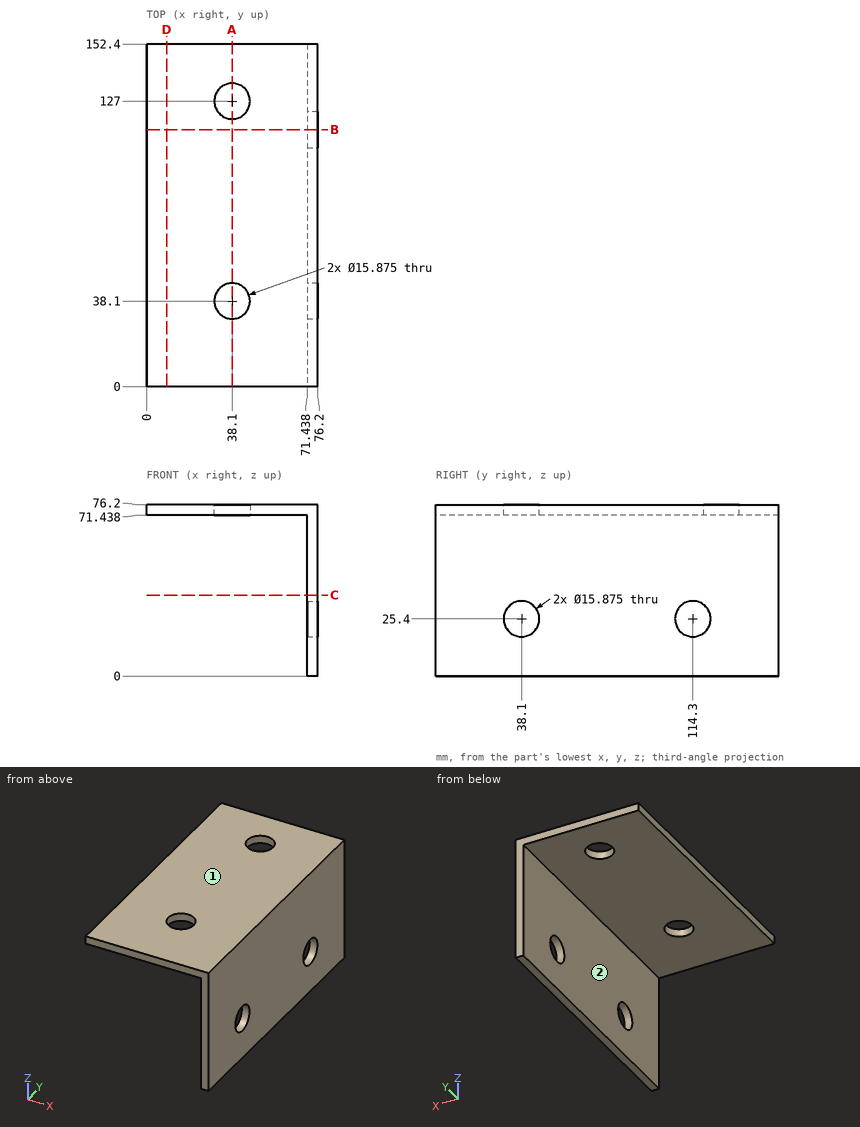
The figure shows three views and two pictorial views of one solid part (mm, origin at its lowest corner). Answer the questions. A direction names the side the tool comes from. Round coordinates to 2 decimals unless told otherwise and drop trailing zeros. Loops run counter-clockwise (first coordinate to the right, second up) from the corner with the lowest first, then second, coordinate; pieces in that order, holes last. Notation, with made-up numbers: (13, -6.5) - (48, -6.5) arc R23 ccw to (48, 30.5) - close; hole circle Ø2 at (-37, 38). An arc over 180 degrees is marked (long way). One line per question, with ' | ' between items. Start each with the question number.
Q1. Section D-D on x = 9 is taken. Give the vertices of the cut face in (y, z).
Q2. Section B-B on y = 114.3 is taken. Give the vertices of the cut face in (x, z).
Q3. Find the intervals of material crossed by L1, parallel to Y at x = 38.1, z = 73.75; L2, parallel to Z at x = 75.1, y = 114.3; L3, parallel to X at y = 15.5, z = 35, in increasing order.
Q4. For the marked faces 1 and 2, determine the directions among +Z, -Z, +X, -X, +Y, -Y from which every point of the face is accessible in a straight line to the end or side of a thin tool.
Q5. Section A-A on x = 38.1 is taken. Give the vertices of the cut face in (y, z).
Q6. Flat-ended cylindrical pins translate along their axes: pin 1 (1.5 mm diameter, centred on y = 20, z = 35.5, fed in from -X); pin 2 (21.5 mm diameter, centred on x = 40, y = 102, fed in from -Z); pin 3 (9.5 mm diameter, centred on y = 114.3, z = 25.4, fed in from -X). Find the tip coordinate at first contact, or state that the pin passes through.
Q7. Section C-C on z = 36 is taken. Give the vertices of the cut face in (x, y).
Established:
1) outline: (0, 71.44) - (152.4, 71.44) - (152.4, 76.2) - (0, 76.2) - close
2) outline: (0, 71.44) - (71.44, 71.44) - (71.44, 33.34) - (76.2, 33.34) - (76.2, 76.2) - (0, 76.2) - close; (71.44, 0) - (76.2, 0) - (76.2, 17.46) - (71.44, 17.46) - close
3) L1: 0 to 30.16, 46.04 to 119.06, 134.94 to 152.4 | L2: 0 to 17.46, 33.34 to 76.2 | L3: 71.44 to 76.2
4) face 1: +Z, +X, -X, +Y, -Y | face 2: -Z, -X, +Y, -Y
5) outline: (0, 71.44) - (30.16, 71.44) - (30.16, 76.2) - (0, 76.2) - close; (46.04, 71.44) - (119.06, 71.44) - (119.06, 76.2) - (46.04, 76.2) - close; (134.94, 71.44) - (152.4, 71.44) - (152.4, 76.2) - (134.94, 76.2) - close
6) pin 1: x = 71.44 | pin 2: z = 71.44 | pin 3: through
7) outline: (71.44, 0) - (76.2, 0) - (76.2, 152.4) - (71.44, 152.4) - close
